from build123d import *

# Parameters (mm, degrees)
SKETCH1_W                        = 57.15
SKETCH1_H                        = 76.2
EXTRUDE1_DEPTH                   = 12.7
F_1_4_CLEARANCE_HOLE1_AT_2_COUNT = 2
F_1_4_CLEARANCE_HOLE1_AT_2_PITCH = 60.325
F_1_4_CLEARANCE_HOLE1_AT_3_COUNT = 2
F_1_4_CLEARANCE_HOLE1_AT_3_PITCH = 38.1
CUT_EXTRUDE2_DEPTH               = 13.7
CHAMFER1_SIZE                    = 1.524


with BuildPart() as part:
    # Sketch1 → Extrude1 (new body)
    with BuildSketch(Plane(origin=(0, 0, 0), x_dir=(0, 0, -1), z_dir=(1, 0, 0))):
        Rectangle(SKETCH1_W, SKETCH1_H)
    extrude(amount=EXTRUDE1_DEPTH)

    # Sketch2 → 1/4 Clearance Hole1 (revolve, cut)
    with BuildSketch(Plane(origin=(12.7, 30.1625, 20.6375), x_dir=(0, 0, -1), z_dir=(0, 1, 0))):
        Polygon((0, 0), (0, 12.7), (4.191, 12.7), (3.57124, 11.987047676), (3.57124, 0.712952324), (4.191, 0), align=None)
    f_1_4_clearance_hole1 = revolve(axis=Axis((19.05, 30.1625, 20.6375), (-1, 0, 0)), mode=Mode.SUBTRACT)

    # 1/4 Clearance Hole1 at 2: 1/4 Clearance Hole1 ×2
    with Locations(*[(0, -i * F_1_4_CLEARANCE_HOLE1_AT_2_PITCH, 0) for i in range(1, F_1_4_CLEARANCE_HOLE1_AT_2_COUNT)]):
        add(f_1_4_clearance_hole1, mode=Mode.SUBTRACT)

    # 1/4 Clearance Hole1 at 3: 1/4 Clearance Hole1 ×2
    with Locations(*[(0, 0, -i * F_1_4_CLEARANCE_HOLE1_AT_3_PITCH) for i in range(1, F_1_4_CLEARANCE_HOLE1_AT_3_COUNT)]):
        add(f_1_4_clearance_hole1, mode=Mode.SUBTRACT)

    # Sketch4 → 3/8-24 Tapped Hole1 (revolve, cut)
    with BuildSketch(Plane(origin=(12.7, 0, -9.525), x_dir=(0, 0, -1), z_dir=(0, 1, 0))):
        Polygon((0, 0), (0, 12.7), (5.3975, 12.7), (4.2164, 11.341299874), (4.2164, 1.358700126), (5.3975, 0), align=None)
    revolve(axis=Axis((19.05, 0, -9.525), (-1, 0, 0)), mode=Mode.SUBTRACT)

    # Sketch7 → Cut-Extrude2 (cut, through all)
    with BuildSketch(Plane(origin=(12.7, 0, 0), x_dir=(0, 0, -1), z_dir=(1, 0, 0))):
        Polygon((-9.525, -38.1), (28.575, 0), (28.575, -38.1), align=None)
    extrude(amount=-CUT_EXTRUDE2_DEPTH, mode=Mode.SUBTRACT)

    # Chamfer1
    chamfer1_edges = [part.edges().sort_by_distance(p)[0] for p in [
        (12.7, 38.1, 0),
        (12.7, 0, 28.575),
        (0, 38.1, 0),
        (0, 19.05, -28.575),
        (12.7, 19.05, -28.575),
        (0, -19.05, -9.525),
        (12.7, -19.05, -9.525),
        (0, -38.1, 19.05),
        (0, 0, 28.575),
        (12.7, -38.1, 19.05),
    ]]
    chamfer(chamfer1_edges, length=CHAMFER1_SIZE)


solid = part.part
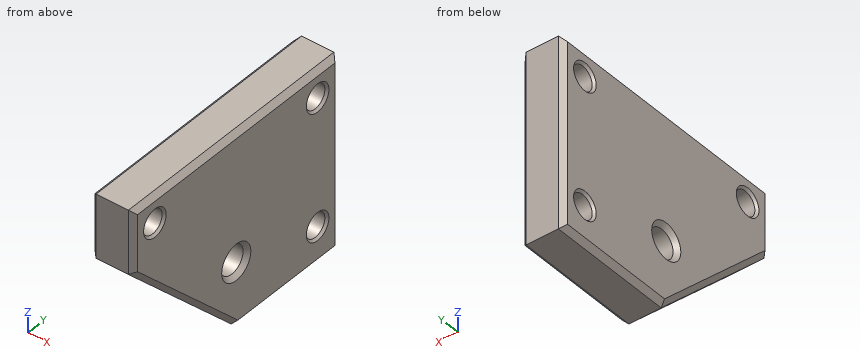
Could you check a few things on this model? Use its own coordinates, in mm. Give positions to 0.01 mm unless a question says otherwise; leave off trailing zeros. Write each loop counter-clockwise with the first axis right and the second up, starting at its lowest first coordinate (ties: lowest second). Pieces come first, ordered by that corner, then holes. Notation, with made-up numbers: (-30.5, 32.25) -> (-8.5, 32.25) arc R20 ccw to (-8.5, 60.25) -> close; hole circle Ø2 at (5, -33.75). An arc over 180 degrees is marked (long way). Answer as CSV lines item,"result". Start each with the question number.
(1) Please list where these lines run through material, in increasing order: line 1 (Y direction, x = 6.5, z = 21.5); line 2 (Z direction, x = 3.5, y = 31.5) (3 decimals); line 3 (Z direction, x = 6, y = 0) (3 decimals).
(2) I'm going to push flat-ended pins straight in: pin 1 Ø3 at (x, z) = (1.5, -17.5) entering from -Y; pin 2 Ø5.5 at (y, z) = (30.16, -17.46) entering from +X. Where does each tip first touch, or does it pass through?
(3) If we section it at B-B, the plane z = 0: Write out the boundary of the cut face in (x, y) (3 decimals), and give its area (3 significant figures).
(4) If we section it at A-A, the plane x = 8.75: Write out the boundary of the cut face in (y, z) (1 decimal).
(5) If we section it at C-C, the plane y = -12.5: Write out the boundary of the cut face in (x, z) (3 decimals), and give its area (3 significant figures).
Answer list:
1,line 1,"-38.1 to -33.63, -26.7 to 26.7, 33.63 to 38.1"
1,line 2,"-28.575 to -20.774, -14.151 to 17.326, 23.949 to 28.575"
1,line 3,"-28.575 to -13.741, -5.309 to 28.575"
2,pin 1,"y = -12.57"
2,pin 2,"through"
3,outline,"(0, -26.42) -> (1.524, -28.575) -> (11.176, -28.575) -> (12.7, -26.42) -> (12.7, 36.576) -> (11.176, 38.1) -> (1.524, 38.1) -> (0, 36.576) -> close"
3,area,"841 mm^2"
4,outline,"(-38.1, 9.5) -> (0, -28.6) -> (38.1, -28.6) -> (38.1, 28.6) -> (-38.1, 28.6) -> close; hole circle Ø7.1 at (-30.2, 20.6); hole circle Ø8.4 at (0, -9.5); hole circle Ø7.1 at (30.2, -17.5); hole circle Ø7.1 at (30.2, 20.6)"
5,outline,"(0, -13.92) -> (1.524, -16.075) -> (11.176, -16.075) -> (12.7, -13.92) -> (12.7, 27.051) -> (11.176, 28.575) -> (1.524, 28.575) -> (0, 27.051) -> close"
5,area,"561 mm^2"
